For this review, take the finished solid that the model builds, in its own axes (mm). Face numbers are marked on the shaded views. A direction names the side the tool comes from. Coordinates: 2 decimals unless noted, no trailing zeros. Write each loop counter-clockwise with the first axis right and the second up, starting at its lowest first coordinate (ties: lowest second). Pieces come first, ordered by that corner, then holes. Notation, with made-up numbers: M -10.75,81 L 10.25,81 A32 ccw 10.25,116 Z; hole C 18.5,-21.75 d6. An arc over 180 degrees is marked long. One line per question, with ' | ' between items.
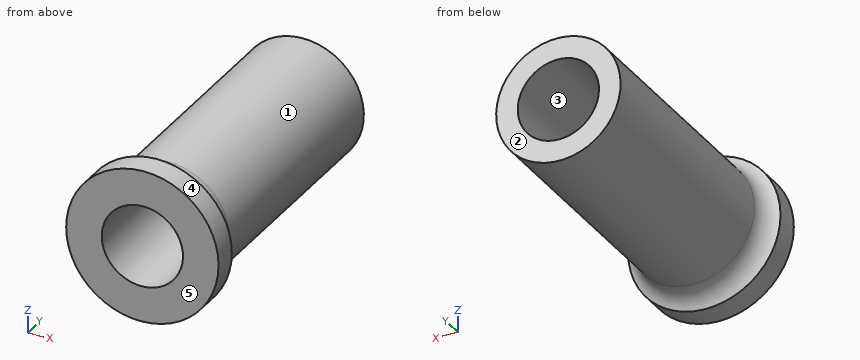
from build123d import *

# Parameters (mm, degrees)
SKETCH1_R           = 2.45
SKETCH1_R_2         = 1.5
BOSS_EXTRUDE1_DEPTH = 11
SKETCH2_R           = 3
BOSS_EXTRUDE2_DEPTH = 1
SKETCH3_R           = 1.6
CUT_EXTRUDE1_DEPTH  = 13.727922061
FILLET2_R           = 1


with BuildPart() as part:
    # Sketch1 → Boss-Extrude1 (new body)
    with BuildSketch(Plane(origin=(0, 0, 0), x_dir=(1, 0, 0), z_dir=(0, 1, 0))):
        with Locations(Location((0, 0, 0), (0, 0, 270))):
            Circle(SKETCH1_R)
        with Locations(Location((0, 0, 0), (0, 0, 270))):
            Circle(SKETCH1_R_2, mode=Mode.SUBTRACT)
    extrude(amount=BOSS_EXTRUDE1_DEPTH)

    # Sketch2 → Boss-Extrude2 (add)
    with BuildSketch(Plane(origin=(0, 0, 0), x_dir=(-1, 0, 0), z_dir=(0, -1, 0))):
        with Locations(Location((0, 0, 0), (0, 0, 90))):
            Circle(SKETCH2_R)
    extrude(amount=BOSS_EXTRUDE2_DEPTH)

    # Sketch3 → Cut-Extrude1 (cut, through all)
    with BuildSketch(Plane(origin=(0, -1, 0), x_dir=(-1, 0, 0), z_dir=(0, -1, 0))):
        with Locations(Location((0, 0, 0), (0, 0, 90))):
            Circle(SKETCH3_R)
    extrude(amount=-CUT_EXTRUDE1_DEPTH, mode=Mode.SUBTRACT)

    # Fillet2
    # the kernel refuses this fillet: 1 mm, written as the material it adds along each edge
    with BuildSketch(Plane(origin=(0, 0, 0), x_dir=(0, 0, 1), z_dir=(-1, 0, 0))) as fillet2_piece_1:
        with BuildLine():
            CenterArc((3.45, 0.893028555), FILLET2_R, 180, 63.25631605)
            Line((2.45, 0.893028555), (2.43, 0.893028555))
            Line((2.43, 0.893028555), (2.43, 0))
            Line((2.43, 0), (2.45, -0.02))
            ThreePointArc((2.45, -0.02), (2.725, -0.02), (2.991, -0.017860571))
            Line((2.991, -0.017860571), (3, 0))
        make_face()
    revolve(axis=Axis((0, 0, 0), (0, 1, 0)))


solid = part.part
1) To check wall thickness, follow line 1 along X through (y, z) = (1.5, 0); line 2 along Z through (x, y) = (0.4, 2). State the ranges of each line that lie inside material, in increasing order. Write a range as [from, to].
Responses:
line 1: [-2.45, -1.6], [1.6, 2.45] | line 2: [-2.42, -1.55], [1.55, 2.42]
2) We need section D-D on y = 0.5. State the section outline as (x, z) points.
Responses:
outline: C 0,0 d5.06; hole C 0,0 d3.2
3) We need section B-B on x = 0. State the section outline as (y, z) points.
Responses:
outline: M -1,-3 L 0,-3 A1 cw 0.89,-2.45 L 11,-2.45 L 11,-1.6 L -1,-1.6 Z; M -1,1.6 L 11,1.6 L 11,2.45 L 0.89,2.45 A1 cw 0,3 L -1,3 Z
4) We need section A-A on z = 0. State the section outline as (x, y) points, then the cut area to 3 significant figures.
Responses:
outline: M -3,-1 L -1.6,-1 L -1.6,11 L -2.45,11 L -2.45,0.89 A1 cw -3,0 Z; M 1.6,-1 L 3,-1 L 3,0 A1 cw 2.45,0.89 L 2.45,11 L 1.6,11 Z | area: 21.8 mm^2
5) The part is to be moulded in two halves that separate along X. For the marked faces 3, 4 and 5, say which applies: +X half, -X half, draft (parallel to the pull), parting line (faces both ways), or undercut.
Responses:
face 3: undercut | face 4: parting line | face 5: draft
6) We need section C-C on y = 9.75. State the section outline as (x, z) points.
Responses:
outline: C 0,0 d4.9; hole C 0,0 d3.2
7) Machinability: for the marked faces 1 and 2, which of the approach directions +Z, -Z, +X, -X, +Y, -Y give a long, thin tool a straight path to every point of the face, cutting with its end or side? Answer none if there is none.
Responses:
face 1: +Y | face 2: +Z, -Z, +X, -X, +Y
